Could you check a few things on this model? Use its own coordinates, in mm. A direction names the side the tool comes from. Round coordinates to 2 decimals unless told otherwise and drop trailing zeros. Loops run counter-clockwise (first coordinate to the right, second up) from the corner with the lowest first, then second, coordinate; pieces in that order, holes last. Notation, with made-up numbers: M 87,66.5 L 101,66.5 A6 ccw 101,72.5 Z; hole C 43,63 d8. An arc over 180 degrees is marked long. Answer in a Markdown table with one row per item.
```python
from build123d import *

# Parameters (mm, degrees)
BOSS_EXTRUDE3_DEPTH = 25.4
BOSS_EXTRUDE4_DEPTH = 4
FILLET2_R           = 10


with BuildPart() as part:
    # Sketch4 → Boss-Extrude3 (new body)
    with BuildSketch(Plane.XY):
        with BuildLine():
            Line((79.118213734, 41.276110426), (-12.893671351, 41.276110426))
            ThreePointArc((-12.893671351, 41.276110426), (-40.393671351, 13.776110426), (-12.893671351, -13.723889574))
            Line((-12.893671351, -13.723889574), (79.118213734, -13.723889574))
            Line((79.118213734, -13.723889574), (79.118213734, 41.276110426))
        make_face()
        with BuildLine():
            Line((-12.472737934, 38.276110426), (76.118213734, 38.276110426))
            Line((76.118213734, 38.276110426), (76.118213734, -10.723889574))
            Line((76.118213734, -10.723889574), (-12.472737934, -10.723889574))
            ThreePointArc((-12.472737934, -10.723889574), (-36.972737934, 13.776110426), (-12.472737934, 38.276110426))
        make_face(mode=Mode.SUBTRACT)
    extrude(amount=BOSS_EXTRUDE3_DEPTH)

    # Sketch6 → Boss-Extrude4 (add)
    with BuildSketch(Plane.XY.offset(25.4)):
        with BuildLine():
            Line((-12.893671351, 41.276110426), (79.118213734, 41.276110426))
            Line((79.118213734, 41.276110426), (79.118213734, -13.723889574))
            Line((79.118213734, -13.723889574), (-12.893671351, -13.723889574))
            ThreePointArc((-12.893671351, -13.723889574), (-40.393671351, 13.776110426), (-12.893671351, 41.276110426))
        make_face()
    extrude(amount=-BOSS_EXTRUDE4_DEPTH)

    # Fillet2
    fillet2_edges = [part.edges().sort_by_distance(p)[0] for p in [
        (-40.393671351, 13.776110426, 25.4),
        (33.112271192, -13.723889574, 25.4),
        (33.112271192, 41.276110426, 25.4),
    ]]
    fillet(fillet2_edges, radius=FILLET2_R)


solid = part.part
```
1) I want a section at C-C, the plane z = 19.25. Please give me the cut outline in (x, y).
Computed:
| item | result |
|---|---|
| outline | M -12.89,-12.95 L 79.12,-12.95 L 79.12,40.51 L -12.89,40.51 A26.73 ccw Z; hole M -12.47,-10.72 L 76.12,-10.72 L 76.12,38.28 L -12.47,38.28 A24.5 ccw Z |
2) I need wall thicknesses on line 1 (Y direction, x = 19, z = 4.25); line 2 (X direction, y = 6.5, z = 8.5); line 3 (Y direction, x = -14, z = 7.5). Which ranges of each line are inside material? Lowest first, please.
Computed:
| item | result |
|---|---|
| line 1 | y = -13.72 to -10.72, 38.28 to 41.28 |
| line 2 | x = -39.41 to -35.87, 76.12 to 79.12 |
| line 3 | y = -13.7 to -10.68, 38.23 to 41.25 |
3) If we mould it in two halves opening along X, with no side actions, what happens to faces 3 (the face through (32.47, 38.27, 22.55)), 4 (the face through (-40.387, 14.381, 7.592)), 5 (the face through (79.118, 13, 13)), 6 (the face through (76.118, 14, 11))? For each: released by +X, released by -X, zero draft, split by the parting line, or undercut.
Computed:
| item | result |
|---|---|
| face 3 | zero draft |
| face 4 | released by -X |
| face 5 | released by +X |
| face 6 | undercut |
4) I want a section at A-A, the plane z = 9. Please give me the cut outline in (x, y).
Computed:
| item | result |
|---|---|
| outline | M -12.89,-13.72 L 79.12,-13.72 L 79.12,41.28 L -12.89,41.28 A27.5 ccw Z; hole M -12.47,-10.72 L 76.12,-10.72 L 76.12,38.28 L -12.47,38.28 A24.5 ccw Z |
5) Which directions (+Z, -Z, +X, -X, +Y, -Y) give clear straight access to the entire face, cutting with the end or side of a thin tool? Please do faces 1 (the face through (20, 14, 21.4)), 2 (the face through (33.756, -10.717, 22.548)).
Computed:
| item | result |
|---|---|
| face 1 | -Z |
| face 2 | +Z, +X, -X, -Y |
6) Will these pins go through, and if not, where does the flat tip stop? P1, Ø24.5, axis at x = 22.5, y = 15.5, coming from the -Z side; P2, Ø6.5, axis at y = 23, z = 13.5, coming from the -X side; P3, Ø1, axis at y = 35.5, z = 7, coming from the -X side.
Computed:
| item | result |
|---|---|
| P1 | stops at z = 21.4 |
| P2 | stops at x = -39.74 |
| P3 | stops at x = -30.38 |
7) I want a section at B-B, the plane x = 10. Please give me the cut outline in (y, z).
Computed:
| item | result |
|---|---|
| outline | M -13.72,0 L -10.72,0 L -10.72,21.4 L 38.28,21.4 L 38.28,0 L 41.28,0 L 41.28,15.4 A10 ccw 31.28,25.4 L -3.72,25.4 A10 ccw -13.72,15.4 Z |
